Could you check a few things on this model? Use its own coordinates, in mm. Face numbers are marked on the shaded views. A direction names the side the tool comes from. Give positions to 0.01 mm unless a question says otherwise; leave off trailing zeros. Write each loop counter-clockwise with the first axis right and the second up, starting at its lowest first coordinate (ties: lowest second). Pieces come first, ordered by that corner, then holes. Notation, with made-up numbers: (36.25, 14.5) - (77.25, 14.5) arc R32 ccw to (77.25, 53.5) - close; hole circle Ø10 at (59.25, 29.25). An arc over 180 degrees is marked (long way). Answer in a Markdown table with one row per item.
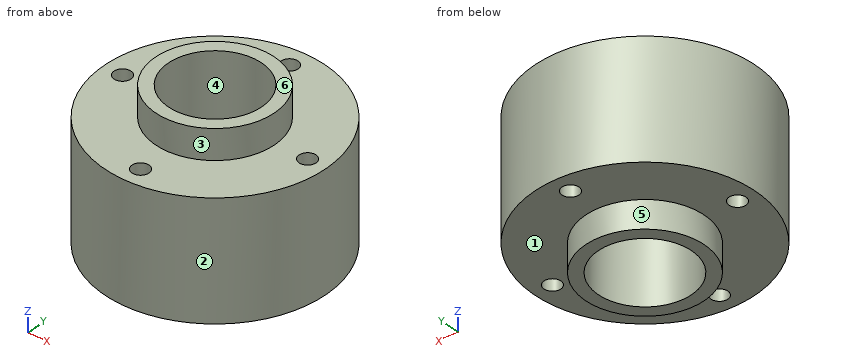
from build123d import *

# Parameters (mm, degrees)
BOSS_EXTRUDE1_START      = -4.5
SKETCH1_R                = 26
SKETCH1_R_2              = 2
SKETCH1_R_3              = 14
BOSS_EXTRUDE1_DEPTH      = 27.531540746
BOSS_EXTRUDE2_DEPTH      = 7
BOSS_EXTRUDE2_DEPTH_BACK = 34
SKETCH3_R                = 14
SKETCH3_R_2              = 11


with BuildPart() as part:
    # Sketch1 → Boss-Extrude1 (new body)
    with BuildSketch(Plane.XY.offset(BOSS_EXTRUDE1_START)):
        Circle(SKETCH1_R)
        with Locations((21.45, 0)):
            Circle(SKETCH1_R_2, mode=Mode.SUBTRACT)
        with Locations((0, -21.45)):
            Circle(SKETCH1_R_2, mode=Mode.SUBTRACT)
        Circle(SKETCH1_R_3, mode=Mode.SUBTRACT)
        with Locations((-21.45, 0)):
            Circle(SKETCH1_R_2, mode=Mode.SUBTRACT)
        with Locations((0, 21.45)):
            Circle(SKETCH1_R_2, mode=Mode.SUBTRACT)
    extrude(amount=-BOSS_EXTRUDE1_DEPTH)

    # Sketch3 → Boss-Extrude2 (add, two sides: drawn at the far end of the back side and taken through both)
    with BuildSketch(Plane.XY.offset(-4.5).offset(-BOSS_EXTRUDE2_DEPTH_BACK)):
        Circle(SKETCH3_R)
        Circle(SKETCH3_R_2, mode=Mode.SUBTRACT)
    extrude(amount=BOSS_EXTRUDE2_DEPTH + BOSS_EXTRUDE2_DEPTH_BACK)


solid = part.part
1) Imagine slicing it at C-C (y = 9.5). List the corners of the cut face in (x, z) for me.
Check values:
| item | result |
|---|---|
| outline | (-24.2, -32.03) - (-10.28, -32.03) - (-10.28, -38.5) - (-5.55, -38.5) - (-5.55, 2.5) - (-10.28, 2.5) - (-10.28, -4.5) - (-24.2, -4.5) - close; (5.55, -38.5) - (10.28, -38.5) - (10.28, -32.03) - (24.2, -32.03) - (24.2, -4.5) - (10.28, -4.5) - (10.28, 2.5) - (5.55, 2.5) - close |
2) Will these pins go through, and if not, where does the flat tip stop? P1, Ø1, axis at x = 11, z = -5, coming from the -Y side; P2, Ø4.5, axis at x = 0, y = -21.45, coming from the -Z side; P3, Ø3.5, axis at x = 21.45, y = 0, coming from the +Z side; P4, Ø2, axis at x = -10.5, z = -19, coming from the -Y side.
Check values:
| item | result |
|---|---|
| P1 | stops at y = -23.79 |
| P2 | stops at z = -32.03 |
| P3 | passes through |
| P4 | stops at y = -24.2 |
3) Imagine slicing it at D-D (z = -11.5). List the corners of the cut face in (x, y) for me.
Check values:
| item | result |
|---|---|
| outline | circle Ø52 at (0, 0); hole circle Ø4 at (-21.45, 0); hole circle Ø22 at (0, 0); hole circle Ø4 at (0, -21.45); hole circle Ø4 at (0, 21.45); hole circle Ø4 at (21.45, 0) |
4) On a 3-axis mill with a long thin cutter (end or side, diameter ignored), from which of +Z, -Z, +X, -X, +Y, -Y can I reach the whole of each face in a straight line? I mean the marked faces 1, 2 and 3. Say none if no direction works.
Check values:
| item | result |
|---|---|
| face 1 | -Z |
| face 2 | +Z, -Z |
| face 3 | +Z |
5) If I drill on line 1 (Y direction, x = 0, z = -18); line 2 (Z direction, x = 20, y = -10); line 3 (X direction, y = 7, z = -17), over which ranges is the centre line in solid material (lowest first)?
Check values:
| item | result |
|---|---|
| line 1 | y = -26 to -23.45, -19.45 to -11, 11 to 19.45, 23.45 to 26 |
| line 2 | z = -32.03 to -4.5 |
| line 3 | x = -25.04 to -8.49, 8.49 to 25.04 |
6) Imagine slicing it at A-A (y = 0). List the corners of the cut face in (x, z) for me, then the cut area to 3 significant figures.
Check values:
| item | result |
|---|---|
| outline | (-26, -32.03) - (-23.45, -32.03) - (-23.45, -4.5) - (-26, -4.5) - close; (-19.45, -32.03) - (-14, -32.03) - (-14, -38.5) - (-11, -38.5) - (-11, 2.5) - (-14, 2.5) - (-14, -4.5) - (-19.45, -4.5) - close; (11, -38.5) - (14, -38.5) - (14, -32.03) - (19.45, -32.03) - (19.45, -4.5) - (14, -4.5) - (14, 2.5) - (11, 2.5) - close; (23.45, -32.03) - (26, -32.03) - (26, -4.5) - (23.45, -4.5) - close |
| area | 687 mm2 |
7) We'd pull the mould along X, two halves only. Please class the marked faces 4, 5 and 6: +X half, -X half, draft (parallel to the pull), parting line (faces both ways), or undercut.
Check values:
| item | result |
|---|---|
| face 4 | undercut |
| face 5 | parting line |
| face 6 | draft |
